Input: part model. Units: mm. Frame: model coordinates. A direction names the side the tool comes from. Coordinates: 2 decimals unless noted, no trailing zeros. Loops run counter-clockwise (first coordinate to the right, second up) from the corner with the lowest first, then second, coordinate; pieces in that order, holes last. Notation, with made-up numbers: M -22.75,60.25 L 15.25,60.25 A8 ccw 15.25,67.25 Z; hole C 56.25,41 d10. An arc over 180 degrees is marked long. Use a Markdown table: item, result. Add a question column.
1. Section C-C on x = -16. Output: boundary loops of the cut face in (y, z) (3 decimals).
2. Section B-B on z = 18.5. Output: boundary loops of the cut face in (x, y).
3. Draft query along Y for faces 1 (the cylindrical face through (-33.15, 9.73, 46.99)), 2 (the cylindrical face through (-1.726, -4.632, 8.476)), 3 (the flat face through (-5, -6, 2)), 4 (the flat face through (-26, -11.5, 25)). Return one class per face: +Y half, -Y half, draft (parallel to the pull), parting line (faces both ways), or undercut.
4. Line query: L1, parallel to Z at x = -16, y = 9.05; L2, parallel to Y at x = -2, z = 40; L3, parallel to Z at x = -16, y = -8.8 (3 decimals). Output: solid intervals per line, ascending. Write a range as [from, to].
5. Section D-D on x = -27. Output: boundary loops of the cut face in (y, z), then the cut area to 3 significant figures.
6. Section A-A on z = 35. Output: boundary loops of the cut face in (x, y), then the cut area to 4 significant figures.
7. Set-up query: faces 5 (the flat face through (-3.5, 0, 25)), 6 (the flat face through (-5, 6, 48)), 7 (the flat face through (-3, -2, 0)), 8 (the cylindrical face through (-16.22, -9.77, 42.07)), 9 (the cylindrical face through (-21.9, 9.8, 29.6)). Return all of +Z, -Z, +X, -X, +Y, -Y with unobstructed straight access to the full face (end or side cutting, diameter ignored); none if empty.
8. Pin query (flat end, axial travel): pin 1 (5 mm diameter, centred on y = 1, z = 39, fed in from -X). Return the tip coordinate at first contact, or that it passes through.
```python
from build123d import *

# Parameters (mm, degrees)
EXTRUDE_1_DEPTH     = 50
CUT_EXTRUDE_START   = -19.5
SKETCH_2_R          = 1.5
CUT_EXTRUDE_1_DEPTH = 70
SKETCH_3_OUTSIDE_W  = 61.218
SKETCH_3_OUTSIDE_H  = 66.218
CUT_EXTRUDE_2_DEPTH = 70
SKETCH_5_R          = 1
CUT_EXTRUDE_5_DEPTH = 10
SKETCH_6_W          = 13
SKETCH_6_H          = 23.5
CUT_EXTRUDE_6_DEPTH = 10
SKETCH_7_R          = 1.65
CUT_EXTRUDE_7_DEPTH = 10
SKETCH_8_R          = 8
CUT_EXTRUDE_8_DEPTH = 10
EXTRUDE_2_DEPTH     = 3.5
EXTRUDE_3_DEPTH     = 3.5


with BuildPart() as part:
    # 草图1 → 凸台-拉伸1 (new body)
    with BuildSketch(Plane.XY):
        Polygon((-45, 11.5), (0, 11.5), (0, -11.5), (-45, -11.5), (-45, -8), (-3.5, -8), (-3.5, 8), (-45, 8), align=None)
    extrude(amount=EXTRUDE_1_DEPTH)

    # 草图2 → 切除-拉伸1 (cut)
    with BuildSketch(Plane.XZ.offset(11.5).offset(CUT_EXTRUDE_START)):
        with Locations((-16, 35)):
            Circle(SKETCH_2_R)
        with Locations((-16, 15)):
            Circle(SKETCH_2_R)
    extrude(amount=-CUT_EXTRUDE_1_DEPTH, mode=Mode.SUBTRACT)

    # 草图3 outside → 切除-拉伸2 (cut)
    with BuildSketch(Plane.XZ.offset(11.5)):
        with Locations((-22.5, 25)):
            Rectangle(SKETCH_3_OUTSIDE_W, SKETCH_3_OUTSIDE_H)
        with BuildLine():
            Line((-36, 10), (-36, 40))
            ThreePointArc((-36, 40), (-33.071067812, 47.071067812), (-26, 50))
            Line((-26, 50), (0, 50))
            Line((0, 50), (0, 0))
            Line((0, 0), (-26, 0))
            ThreePointArc((-26, 0), (-33.071067812, 2.928932188), (-36, 10))
        make_face(mode=Mode.SUBTRACT)
    extrude(amount=-CUT_EXTRUDE_2_DEPTH, mode=Mode.SUBTRACT)

    # 草图5 → 切除-拉伸5 (cut)
    with BuildSketch(Plane.XZ.offset(11.5)):
        with Locations((-16, 43.045)):
            Circle(SKETCH_5_R)
        with Locations((-16, 15.375)):
            Circle(SKETCH_5_R)
    extrude(amount=-CUT_EXTRUDE_5_DEPTH, mode=Mode.SUBTRACT)

    # 草图6 → 切除-拉伸6 (cut)
    with BuildSketch(Plane.XZ.offset(11.5)):
        with Locations((-16, 29.21)):
            Rectangle(SKETCH_6_W, SKETCH_6_H)
    extrude(amount=-CUT_EXTRUDE_6_DEPTH, mode=Mode.SUBTRACT)

    # 草图7 → 切除-拉伸7 (cut)
    with BuildSketch(Plane(origin=(0, 0, 0), x_dir=(0, 0, -1), z_dir=(1, 0, 0))):
        with Locations((-10, 4)):
            Circle(SKETCH_7_R)
        with Locations((-40, 4)):
            Circle(SKETCH_7_R)
        with Locations((-10, -4)):
            Circle(SKETCH_7_R)
        with Locations((-40, -4)):
            Circle(SKETCH_7_R)
    extrude(amount=-CUT_EXTRUDE_7_DEPTH, mode=Mode.SUBTRACT)

    # 草图8 → 切除-拉伸8 (cut)
    with BuildSketch(Plane(origin=(0, 11.5, 0), x_dir=(1, 0, 0), z_dir=(0, 1, 0))):
        with Locations((-16, -35)):
            Circle(SKETCH_8_R)
    extrude(amount=-CUT_EXTRUDE_8_DEPTH, mode=Mode.SUBTRACT)

    # 草图9 → 凸台-拉伸2 (add)
    with BuildSketch(Plane(origin=(0, 0, 0), x_dir=(-1, 0, 0), z_dir=(0, 0, -1))):
        Polygon((3.5, 4.5), (3.5, 8), (7, 8), align=None)
        Polygon((3.5, -8), (7, -8), (3.5, -4.5), align=None)
    extrude(amount=-EXTRUDE_2_DEPTH)

    # 草图10 → 凸台-拉伸3 (add)
    with BuildSketch(Plane.XY.offset(50)):
        Polygon((-3.5, 8), (-7, 8), (-3.5, 4.5), align=None)
        Polygon((-3.5, -8), (-3.5, -4.5), (-7, -8), align=None)
    extrude(amount=-EXTRUDE_3_DEPTH)


solid = part.part
```
Answers below:
| question | item | result |
|---|---|---|
| 1 | outline | M -11.5,0 L -8,0 L -8,14.375 L -11.5,14.375 Z; M -11.5,16.375 L -8,16.375 L -8,17.46 L -11.5,17.46 Z; M -11.5,40.96 L -8,40.96 L -8,42.045 L -11.5,42.045 Z; M -11.5,44.045 L -8,44.045 L -8,50 L -11.5,50 Z; M 8,0 L 11.5,0 L 11.5,13.5 L 8,13.5 Z; M 8,16.5 L 11.5,16.5 L 11.5,27 L 8,27 Z; M 8,43 L 11.5,43 L 11.5,50 L 8,50 Z |
| 2 | outline | M -36,-11.5 L -22.5,-11.5 L -22.5,-8 L -36,-8 Z; M -36,8 L -3.5,8 L -3.5,-8 L -9.5,-8 L -9.5,-11.5 L 0,-11.5 L 0,11.5 L -36,11.5 Z |
| 3 | face 1 | draft |
| 3 | face 2 | undercut |
| 3 | face 3 | undercut |
| 3 | face 4 | -Y half |
| 4 | L1 | z = [0, 13.5], [16.5, 27], [43, 50] |
| 4 | L2 | y = [-11.5, -5.65], [-2.35, 2.35], [5.65, 11.5] |
| 4 | L3 | z = [0, 14.375], [16.375, 17.46], [40.96, 42.045], [44.045, 50] |
| 5 | outline | M -11.5,0.05 L -8,0.05 L -8,49.95 L -11.5,49.95 Z; M 8,0.05 L 11.5,0.05 L 11.5,49.95 L 8,49.95 Z |
| 5 | area | 349 mm² |
| 6 | outline | M -36,-11.5 L -22.5,-11.5 L -22.5,-8 L -36,-8 Z; M -36,8 L -24,8 L -24,11.5 L -36,11.5 Z; M -9.5,-11.5 L 0,-11.5 L 0,11.5 L -8,11.5 L -8,8 L -3.5,8 L -3.5,-8 L -9.5,-8 Z |
| 6 | area | 206.5 mm² |
| 7 | face 5 | -X |
| 7 | face 6 | +Z, -Z, -X |
| 7 | face 7 | -Z, +X, -X, +Y, -Y |
| 7 | face 8 | -Y |
| 7 | face 9 | +Y |
| 8 | pin 1 | stops at x = -3.5 |
